```python
from build123d import *

# Parameters (mm, degrees)
SKETCH2_R                = 25
BOSS_EXTRUDE1_DEPTH      = 60
SKETCH3_R                = 50
BOSS_EXTRUDE2_DEPTH      = 5
CHAMFER1_SIZE            = 2
SKETCH4_R                = 2.5
CUT_EXTRUDE1_DEPTH       = 144.614066163
CIRPATTERN1_COUNT        = 7
MIRROR1_COPY_1_SKETCH_R  = 2.5
MIRROR1_COPY_1_DEPTH     = 144.614066163
MIRROR1_COPY_2_SKETCH_R  = 2.5
MIRROR1_COPY_2_DEPTH     = 144.614066163
MIRROR1_COPY_3_SKETCH_R  = 2.5
MIRROR1_COPY_3_DEPTH     = 144.614066163
MIRROR1_COPY_4_SKETCH_R  = 2.5
MIRROR1_COPY_4_DEPTH     = 144.614066163
MIRROR1_COPY_5_SKETCH_R  = 2.5
MIRROR1_COPY_5_DEPTH     = 144.614066163
MIRROR1_COPY_6_SKETCH_R  = 2.5
MIRROR1_COPY_6_DEPTH     = 144.614066163
CHAMFER1_OF_MIRROR1_SIZE = 2


with BuildPart() as part:
    # Sketch2 → Boss-Extrude1 (new, symmetric)
    with BuildSketch(Plane.XY):
        Circle(SKETCH2_R)
    extrude(amount=BOSS_EXTRUDE1_DEPTH, both=True)

    # Sketch3 → Boss-Extrude2 (add)
    with BuildSketch(Plane.XY.offset(60)):
        Circle(SKETCH3_R)
    boss_extrude2 = extrude(amount=BOSS_EXTRUDE2_DEPTH)

    # Chamfer1
    chamfer1_edges = [part.edges().sort_by_distance(p)[0] for p in [
        (-50, 0, 65),
    ]]
    chamfer(chamfer1_edges, length=CHAMFER1_SIZE)

    # Sketch4 → Cut-Extrude1 (cut, through all)
    with BuildSketch(Plane.XY.offset(65)):
        with Locations((0, 37.5)):
            Circle(SKETCH4_R)
    cut_extrude1 = extrude(amount=-CUT_EXTRUDE1_DEPTH, mode=Mode.SUBTRACT)

    # CirPattern1: Cut-Extrude1 ×7 about axis
    cirpattern1_axis = Axis((0, 0, 0), (0, 0, 1))
    for i in range(1, CIRPATTERN1_COUNT):
        add(cut_extrude1.rotate(cirpattern1_axis, i * 360 / CIRPATTERN1_COUNT), mode=Mode.SUBTRACT)

    # Sketch6 → CBORE for #12 Binding Head Machine Screw1 (revolve, cut)
    with BuildSketch(Plane(origin=(0, 0, 65), x_dir=(0, -1, 0), z_dir=(1, 0, 0))):
        Polygon((0, 0), (0, 130), (2.8956, 130), (2.8956, 3.5814), (5.95376, 3.5814), (5.95376, 0.635), (6.58876, 0), align=None)
    cbore_for_12_binding_head_machine_screw = revolve(axis=Axis((0, 0, 71.35), (0, 0, -1)), mode=Mode.SUBTRACT)

    # Mirror1: Boss-Extrude2, Cut-Extrude1, CBORE for #12 Binding Head Machine Screw1 across plane
    add(boss_extrude2.mirror(Plane.XY))
    add(cut_extrude1.mirror(Plane.XY), mode=Mode.SUBTRACT)
    add(cbore_for_12_binding_head_machine_screw.mirror(Plane.XY), mode=Mode.SUBTRACT)

    # Mirror1 copy 1 sketch → Mirror1 copy 1 (cut, through all)
    with BuildSketch(Plane(origin=(0, 0, -65), x_dir=(0.6234898018587336, 0.7818314824680298, 0), z_dir=(0, 0, -1))):
        with Locations((0, -37.5)):
            Circle(MIRROR1_COPY_1_SKETCH_R)
    extrude(amount=-MIRROR1_COPY_1_DEPTH, mode=Mode.SUBTRACT)

    # Mirror1 copy 2 sketch → Mirror1 copy 2 (cut, through all)
    with BuildSketch(Plane(origin=(0, 0, -65), x_dir=(-0.22252093395631434, 0.9749279121818236, 0), z_dir=(0, 0, -1))):
        with Locations((0, -37.5)):
            Circle(MIRROR1_COPY_2_SKETCH_R)
    extrude(amount=-MIRROR1_COPY_2_DEPTH, mode=Mode.SUBTRACT)

    # Mirror1 copy 3 sketch → Mirror1 copy 3 (cut, through all)
    with BuildSketch(Plane(origin=(0, 0, -65), x_dir=(-0.900968867902419, 0.43388373911755823, 0), z_dir=(0, 0, -1))):
        with Locations((0, -37.5)):
            Circle(MIRROR1_COPY_3_SKETCH_R)
    extrude(amount=-MIRROR1_COPY_3_DEPTH, mode=Mode.SUBTRACT)

    # Mirror1 copy 4 sketch → Mirror1 copy 4 (cut, through all)
    with BuildSketch(Plane(origin=(0, 0, -65), x_dir=(-0.9009688679024191, -0.433883739117558, 0), z_dir=(0, 0, -1))):
        with Locations((0, -37.5)):
            Circle(MIRROR1_COPY_4_SKETCH_R)
    extrude(amount=-MIRROR1_COPY_4_DEPTH, mode=Mode.SUBTRACT)

    # Mirror1 copy 5 sketch → Mirror1 copy 5 (cut, through all)
    with BuildSketch(Plane(origin=(0, 0, -65), x_dir=(-0.2225209339563137, -0.9749279121818237, 0), z_dir=(0, 0, -1))):
        with Locations((0, -37.5)):
            Circle(MIRROR1_COPY_5_SKETCH_R)
    extrude(amount=-MIRROR1_COPY_5_DEPTH, mode=Mode.SUBTRACT)

    # Mirror1 copy 6 sketch → Mirror1 copy 6 (cut, through all)
    with BuildSketch(Plane(origin=(0, 0, -65), x_dir=(0.6234898018587334, -0.7818314824680299, 0), z_dir=(0, 0, -1))):
        with Locations((0, -37.5)):
            Circle(MIRROR1_COPY_6_SKETCH_R)
    extrude(amount=-MIRROR1_COPY_6_DEPTH, mode=Mode.SUBTRACT)

    # Chamfer1 of Mirror1
    chamfer1_of_mirror1_edges = [part.edges().sort_by_distance(p)[0] for p in [
        (-50, 0, -65),
    ]]
    chamfer(chamfer1_of_mirror1_edges, length=CHAMFER1_OF_MIRROR1_SIZE)


solid = part.part
```
Source: CAD feature listing. Evaluate the final solid. Frame: model axes, mm. A direction names the side the tool comes from. Coordinates: 2 decimals unless noted, no trailing zeros. Loops run counter-clockwise (first coordinate to the right, second up) from the corner with the lowest first, then second, coordinate; pieces in that order, holes last. Notation, with made-up numbers: M 2,59.25 L 36,59.25 A21 ccw 36,93.25 Z; hole C 46.5,69 d3. An arc over 180 degrees is marked long. Use a Markdown table: item, result. Add a question column.
Q1. Access query for faces 5 (the flat face through (-22.9, -10.4, 60)), 6 (the cylindrical face through (39.06, -8.36, -62.54)), 7 (the cylindrical face through (-5.9, 0.8, -62.9)), 8 (the flat face through (-1, 3, 61.419)). Directions: +Z, -Z, +X, -X, +Y, -Y. A direction counts if a zero-diameter tool reaches every point of the face in a straight line with its end or side. Return the directions, or none.
Q2. First-contact query: pin 1 (4 mm diameter, centred on x = -36.56, y = -8.34, fed in from -Z); pin 2 (8 mm diameter, centred on x = 7.5, z = -45.5, fed in from +Y); pin 3 (3 mm diameter, centred on y = 15.5, z = 10.5, fed in from -X); pin 4 (6.5 mm diameter, centred on x = 0, y = 0, fed in from -Z). Flat tips, straight axial feed; report the tip coordinate or a pass-through.
Q3. Section query B-B, the plane x = 0. State how many separate pieces and enclosed holes the cut face has, and give its area (3 significant figures).
Q4. Draft query along Z for faces 1 (the cylindrical face through (23.846, 7.509, 0.84)), 2 (the flat face through (-1, 3, -61.419)), 3 (the flat face through (-1, -10, 65)), 4 (the cylindrical face through (2.827, 0.628, -0.86)). Return one class per face: pulls with the +Z half, pulls with the -Z half, needs draft (parallel to the pull), parting line crosses it, or undercut.
Q5. Section query C-C, the plane z = 18. Return loops of the section in (x, y), and give its area (3 significant figures).
Q6. Material intervals for L1, parallel to Z at x = 21, y = -42; L2, parallel to Y at x = 0, z = 25; L3, parallel to X at y = -16.5, z = -32.5, sorted ascending.
Result:
| question | item | result |
|---|---|---|
| 1 | face 5 | none |
| 1 | face 6 | +Z, -Z |
| 1 | face 7 | -Z |
| 1 | face 8 | +Z |
| 2 | pin 1 | passes through |
| 2 | pin 2 | stops at y = 24.75 |
| 2 | pin 3 | stops at x = -20.71 |
| 2 | pin 4 | stops at z = -61.42 |
| 3 | separate pieces | 4 |
| 3 | enclosed holes | 0 |
| 3 | area | 6,140 mm2 |
| 4 | face 1 | undercut |
| 4 | face 2 | pulls with the -Z half |
| 4 | face 3 | pulls with the +Z half |
| 4 | face 4 | needs draft |
| 5 | outline | C 0,0 d50; hole C 0,0 d5.79 |
| 5 | area | 1,940 mm2 |
| 6 | L1 | z = -65 to -60, 60 to 65 |
| 6 | L2 | y = -25 to -2.9, 2.9 to 25 |
| 6 | L3 | x = -18.78 to 18.78 |
